Read the model definition and answer for the solid it produces. Units are mm, in the model's axes. A direction names the side the tool comes from. Give positions to 0.01 mm unless a question says otherwise; leave off trailing zeros. Loops run counter-clockwise (first coordinate to the right, second up) from the corner with the lowest first, then second, coordinate; pieces in that order, holes last.
(1) Which of the six approach directions +Z, -Z, +X, -X, +Y, -Y give full straight-line access (tool end or side, diameter ignored) to faces 1 (the face through (0, -21, 9)), 2 (the face through (0, -2, -9))?
(2) Determine the mould class of faces 3 (the face through (-10, -13.6, 9.3)), 4 (the face through (-7.6, -2, -6.2)), 5 (the face through (0, -4, 0)) for opening direction X: pulls with the +X half, pulls with the -X half, needs draft (parallel to the pull), parting line crosses it, or undercut.
(3) Find section D-D, the plane y = -25.5. Write down the section's boundary in (x, z).
(4) Find section B-B, the plane z = 5. Write down the section's boundary in (x, y), then the cut area to 3 significant figures.
(5) Find section A-A, the plane x = -6. Write down the section's boundary in (y, z), then the cut area to 3 significant figures.
(6) Each of these flat-tipped pins is pushed along its axis until it touches: P1, Ø2.5, axis at x = 6, z = -5, coming from the -Y side; P2, Ø6.5, axis at x = -6, z = -5, coming from the -Y side. Where does it stop, or does it pass through?
(7) Straight lines are drawn through the part: probe 1 along Z at (x, y) = (-6, -1.65); probe 2 along Y at (x, z) = (0.75, -0.75); probe 3 along Z at (x, y) = (-4.75, -20). For each, find the intervals that lie inside material, in ascending order.
(8) Find section C-C, the plane x = 1.25. Write down the section's boundary in (y, z).
```python
from build123d import *

# Parameters (mm, degrees)
F0_W     = 20
F0_H     = 22
F0_R     = 2
F1_DEPTH = 4
F2_W     = 20
F2_H     = 4
F3_DEPTH = 35


with BuildPart() as f1:
    # F0 (on Front) → F1 (new body)
    with BuildSketch(Plane.XZ):
        with Locations((0, 2)):
            Rectangle(F0_W, F0_H)
        with Locations((-6, -5)):
            Circle(F0_R, mode=Mode.SUBTRACT)
        with Locations((6, -5)):
            Circle(F0_R, mode=Mode.SUBTRACT)
        with Locations((-6, 5)):
            Circle(F0_R, mode=Mode.SUBTRACT)
        with Locations((6, 5)):
            Circle(F0_R, mode=Mode.SUBTRACT)
    extrude(amount=F1_DEPTH)

    # F2 (on face) → F3 (join)
    with BuildSketch(Plane.XZ.offset(4)):
        with Locations((0, 11)):
            Rectangle(F2_W, F2_H)
    extrude(amount=F3_DEPTH)


solid = f1.part
```
Entries:
1. face 1: -Z, +X, -X, -Y
1. face 2: -Z, +X, -X, +Y, -Y
2. face 3: pulls with the -X half
2. face 4: undercut
2. face 5: needs draft
3. outline: (-10, 9) - (10, 9) - (10, 13) - (-10, 13) - close
4. outline: (-10, -4) - (-8, -4) - (-8, 0) - (-10, 0) - close; (-4, -4) - (4, -4) - (4, 0) - (-4, 0) - close; (8, -4) - (10, -4) - (10, 0) - (8, 0) - close
4. area: 48.0 mm2
5. outline: (-39, 9) - (-4, 9) - (-4, 7) - (0, 7) - (0, 13) - (-39, 13) - close; (-4, -9) - (0, -9) - (0, -7) - (-4, -7) - close; (-4, -3) - (0, -3) - (0, 3) - (-4, 3) - close
5. area: 196 mm2
6. P1: passes through
6. P2: stops at y = -4
7. probe 1: z = -9 to -7, -3 to 3, 7 to 13
7. probe 2: y = -4 to 0
7. probe 3: z = 9 to 13
8. outline: (-39, 9) - (-4, 9) - (-4, -9) - (0, -9) - (0, 13) - (-39, 13) - close
